For this review, use the dimensioned drawing (mm, ordinates from the lowest corner) and the shaded views. A direction names the side the tool comes from. Coordinates: 2 decimals unless noted, no trailing zeros. Loops run counter-clockwise (first coordinate to the right, second up) from the corner with the lowest first, then second, coordinate; pieces in that order, holes last. Notation, with made-up numbers: M 54,-25.5 L 92,-25.5 A11 ccw 92,-11.5 Z; hole C -34,27 d5. An arc over 180 degrees is marked long. Write item = value, one per line. Start each with the question number.
Q1. We need section D-D on z = 8.5. Give the boundary of the cut face in (x, y).
Q2. Mouldability with a two-part tool opening along X and no side actions: class the marked faces 1, 2 and 3 as released by +X, released by -X, zero draft, split by the parting line, or undercut.
Q3. For the marked faces 4, 5 and 6, list the 3-axis set-ups (+Z, -Z, +X, -X, +Y, -Y) from which the entire face can be reached by the end or side of a thin tool; tool diameter is ignored.
Q4. We need section A-A on z = 4.5. Give the boundary of the cut face in (x, y).
Q5. Clearance check with a flat-ended pin moving along its axis: pin 1 Ø0.8 at (x, y) = (4, 4) entering from -Z (1 decimal). State where the tip first meets the part, or that it passes through.
Q6. Wall thickness on probe 1 along X at (y, z) = (1.75, 7.75); probe 2 along Z at (x, y) = (0.5, 2.5) (1 decimal): over which ranges is each line inside the solid? List them lowest first.
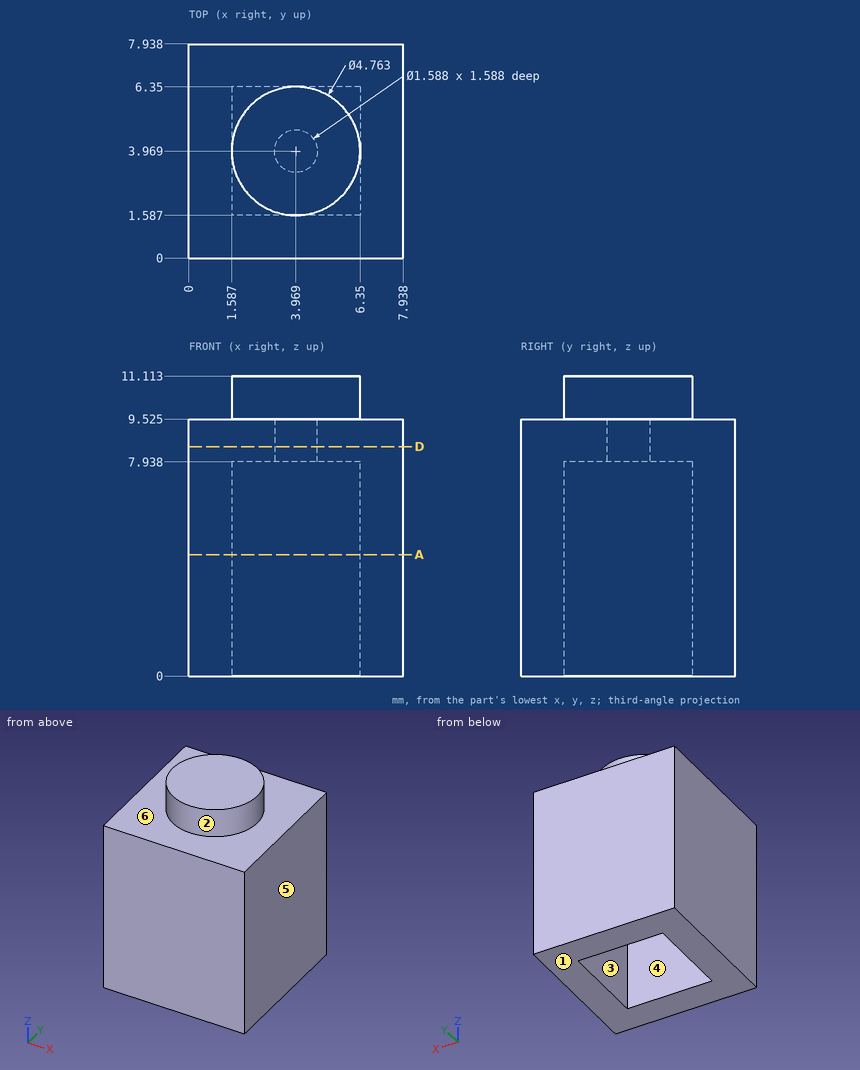
Returned:
q1.outline = M 0,0 L 7.94,0 L 7.94,7.94 L 0,7.94 Z; hole C 3.97,3.97 d1.59
q2.face_1 = zero draft
q2.face_2 = split by the parting line
q2.face_3 = undercut
q3.face_4 = -Z
q3.face_5 = +Z, -Z, +X, +Y, -Y
q3.face_6 = +Z
q4.outline = M 0,0 L 7.94,0 L 7.94,7.94 L 0,7.94 Z; hole M 1.59,1.59 L 6.35,1.59 L 6.35,6.35 L 1.59,6.35 Z
q5.pin_1 = 9.5
q6.probe_1 = 0 to 1.59, 6.35 to 7.94
q6.probe_2 = 0 to 9.5
